Here's the drawing with two shaded views (mm, measured from the low corner). I have some questions. Give positions to 0.01 mm unless a question says otherwise; leave off trailing zeros. Write each loop counter-clockwise with the first axis right and the second up, starting at its lowest first coordinate (ties: lowest second). Pieces come first, ordered by that corner, then holes.
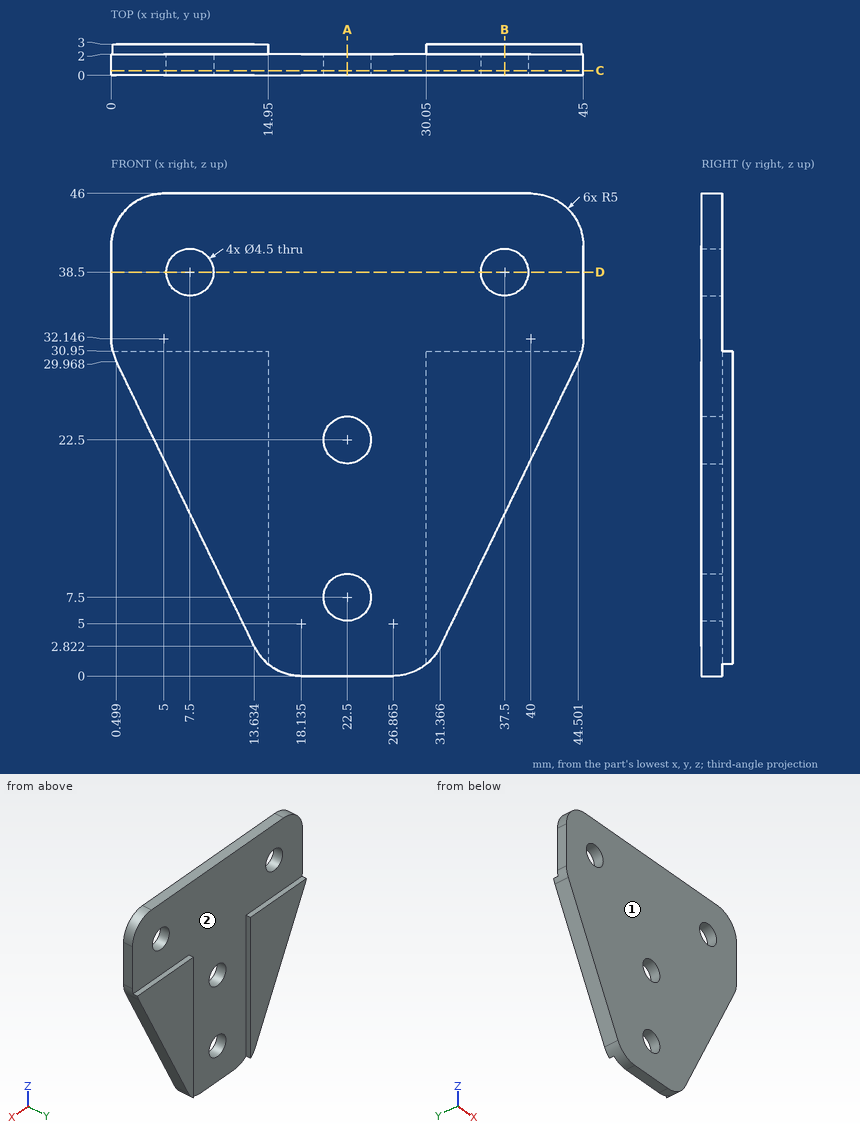
1) Suppose I cut it at A-A on x = 22.5. Write out the boundary of the cut face in (y, z).
Values follow:
outline: (0, 0) - (2, 0) - (2, 5.25) - (0, 5.25) - close; (0, 9.75) - (2, 9.75) - (2, 20.25) - (0, 20.25) - close; (0, 24.75) - (2, 24.75) - (2, 46) - (0, 46) - close
2) Suppose I cut it at C-C on y = 0.45. State how many separate pieces and enclosed holes the cut face has, plus the area to 3 significant figures.
Values follow:
separate pieces: 1
enclosed holes: 4
area: 1,530 mm2
3) For pin 1 Ø0.8 at (y, z) = (2.5, 12) entering from +X; pin 2 Ø0.5 at (x, y) = (36.5, 2.5) entering from +Z; pin 3 Ø1.1 at (y, z) = (2.5, 15.5) entering from -X, each with a flat end and sliding along its axis, tell me the tip position at first contact or that it passes through.
Values follow:
pin 1: stops at x = 36
pin 2: stops at z = 30.95
pin 3: stops at x = 7.23
4) Suppose I cut it at D-D on z = 38.5. Write out the boundary of the cut face in (x, y).
Values follow:
outline: (0, 0) - (5.25, 0) - (5.25, 2) - (0, 2) - close; (9.75, 0) - (35.25, 0) - (35.25, 2) - (9.75, 2) - close; (39.75, 0) - (45, 0) - (45, 2) - (39.75, 2) - close
5) Suppose I cut it at B-B on x = 37.5. Write out the boundary of the cut face in (y, z).
Values follow:
outline: (0, 15.5) - (3, 15.5) - (3, 30.95) - (2, 30.95) - (2, 36.25) - (0, 36.25) - close; (0, 40.75) - (2, 40.75) - (2, 46) - (0, 46) - close
6) Please list where these lines run through material, in increasing order: L1, parallel to X at y = 1.1, z = 38.5; L2, parallel to Z at x = 22.5, y = 1.15; L3, parallel to Y at x = 17, z = 23.
Values follow:
L1: x = 0 to 5.25, 9.75 to 35.25, 39.75 to 45
L2: z = 0 to 5.25, 9.75 to 20.25, 24.75 to 46
L3: y = 0 to 2
7) If we mould it in two halves opening along X, with no side actions, what happens to the marked faces 1 and 2? For each: +X half, -X half, draft (parallel to the pull), parting line (faces both ways), or undercut.
Values follow:
face 1: draft
face 2: undercut
